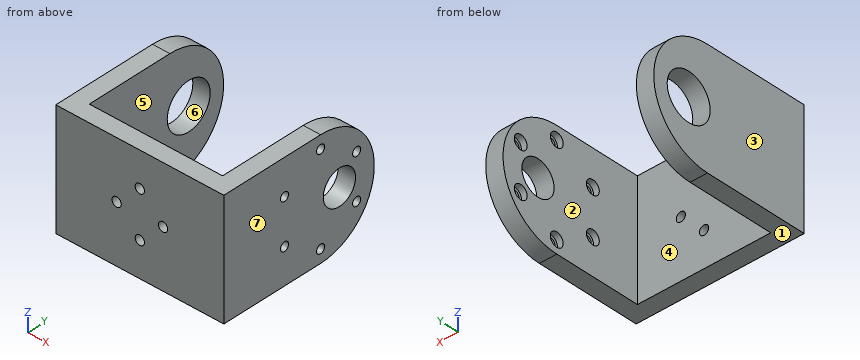
```python
from build123d import *

# Parameters (mm, degrees)
BOSS_EXTRUDE2_DEPTH         = 2
BOSS_EXTRUDE2_DEPTH_BACK    = 4
SKETCH2_W                   = 50
SKETCH2_H                   = 40
BOSS_EXTRUDE3_DEPTH         = 4
BOSS_EXTRUDE3_DEPTH_BACK    = 2
BOSS_EXTRUDE4_DEPTH         = 4
BOSS_EXTRUDE4_DEPTH_BACK    = 2
CUT_EXTRUDE1_DEPTH          = 10
CUT_EXTRUDE1_DEPTH_BACK     = 92
SKETCH7_R                   = 1.5
SKETCH7_R_2                 = 6
SKETCH8_R                   = 3
CUT_EXTRUDE2_DEPTH          = 92
Y_KSEKLIK_EKSTR_ZYON2_DEPTH = 6
SKETCH9_W                   = 11
SKETCH9_H                   = 6
BOSS_EXTRUDE5_DEPTH         = 40
SKETCH10_W                  = 7
SKETCH10_H                  = 40
CUT_EXTRUDE3_DEPTH          = 10
IZIM8_R                     = 2.395734713
KES_EKSTR_ZYON2_DEPTH       = 48
Y_KSEKLIK_EKSTR_ZYON3_DEPTH = 6
IZIM10_R                    = 8
KES_EKSTR_ZYON3_DEPTH       = 6
IZIM11_R                    = 1.6
KES_EKSTR_ZYON5_DEPTH       = 10
IZIM13_R                    = 3.884194159
Y_KSEKLIK_EKSTR_ZYON4_DEPTH = 6


with BuildPart() as part:
    # Sketch2 → Boss-Extrude2 (new, two sides: drawn at the far end of the back side and taken through both)
    with BuildSketch(Plane(origin=(0, 0, 0), x_dir=(1, 0, 0), z_dir=(0, 1, 0)).offset(-BOSS_EXTRUDE2_DEPTH_BACK)):
        with Locations((3.5, 11.198529412)):
            Rectangle(SKETCH2_W, SKETCH2_H)
    extrude(amount=BOSS_EXTRUDE2_DEPTH + BOSS_EXTRUDE2_DEPTH_BACK)

    # Sketch4 → Boss-Extrude3 (add, two sides: drawn at the far end of the back side and taken through both)
    with BuildSketch(Plane.ZY.offset(21.5).offset(-BOSS_EXTRUDE3_DEPTH_BACK)):
        with BuildLine():
            Line((8.801470588, 2), (-31.198529412, 2))
            Line((-31.198529412, 2), (-31.198529412, 32))
            ThreePointArc((-31.198529412, 32), (-11.198529412, 52), (8.801470588, 32))
            Line((8.801470588, 32), (8.801470588, 2))
        make_face()
    extrude(amount=BOSS_EXTRUDE3_DEPTH + BOSS_EXTRUDE3_DEPTH_BACK)

    # Sketch5 → Boss-Extrude4 (add, two sides: drawn at the far end of the back side and taken through both)
    with BuildSketch(Plane(origin=(28.5, 0, 0), x_dir=(0, 0, -1), z_dir=(1, 0, 0)).offset(-BOSS_EXTRUDE4_DEPTH_BACK)):
        with BuildLine():
            Line((-8.801470588, -4), (31.198529412, -4))
            Line((31.198529412, -4), (31.198529412, 32))
            ThreePointArc((31.198529412, 32), (11.198529412, 52), (-8.801470588, 32))
            Line((-8.801470588, 32), (-8.801470588, -4))
        make_face()
    extrude(amount=BOSS_EXTRUDE4_DEPTH + BOSS_EXTRUDE4_DEPTH_BACK)

    # Sketch7 → Cut-Extrude1 (cut, two sides: drawn at the far end of the back side and taken through both)
    with BuildSketch(Plane.ZY.offset(21.5).offset(-CUT_EXTRUDE1_DEPTH_BACK)):
        with Locations(Location((4.301470588, 32, 0), (0, 0, 180))):
            Circle(SKETCH7_R)
        with Locations(Location((-3.448529412, 18.576606241, 0), (0, 0, 180))):
            Circle(SKETCH7_R)
        with Locations(Location((-18.948529412, 18.576606241, 0), (0, 0, 180))):
            Circle(SKETCH7_R)
        with Locations(Location((-26.698529412, 32, 0), (0, 0, 180))):
            Circle(SKETCH7_R)
        with Locations(Location((-18.948529412, 45.423393759, 0), (0, 0, 180))):
            Circle(SKETCH7_R)
        with Locations(Location((-3.448529412, 45.423393759, 0), (0, 0, 180))):
            Circle(SKETCH7_R)
        with Locations(Location((-11.198529412, 39, 0), (0, 0, 180))):
            Circle(SKETCH7_R_2)
    extrude(amount=CUT_EXTRUDE1_DEPTH + CUT_EXTRUDE1_DEPTH_BACK, mode=Mode.SUBTRACT)

    # Sketch8 → Cut-Extrude2 (cut)
    with BuildSketch(Plane(origin=(0, 2, 0), x_dir=(1, 0, 0), z_dir=(0, 1, 0))):
        with Locations(Location((3.5, 11.198529412, 0), (0, 0, 270))):
            Circle(SKETCH8_R)
    extrude(amount=-CUT_EXTRUDE2_DEPTH, mode=Mode.SUBTRACT)

    # Çizim4 → Yükseklik-Ekstrüzyon2 (add)
    with BuildSketch(Plane(origin=(0, 2, 0), x_dir=(1, 0, 0), z_dir=(0, 1, 0))):
        with BuildLine():
            ThreePointArc((6.5, 11.198529412), (6.499830675, 11.230402947), (6.499322719, 11.262272884))
            Line((6.499322719, 11.262272884), (6, 11.262272884))
            Line((6, 11.262272884), (6, 9.540217017))
            ThreePointArc((6, 9.540217017), (6.372281323, 10.332504008), (6.5, 11.198529412))
        make_face()
        with BuildLine():
            Line((6, 11.262272884), (6.499322719, 11.262272884))
            ThreePointArc((6.499322719, 11.262272884), (6.36291811, 12.095022522), (6, 12.856841807))
            Line((6, 12.856841807), (6, 11.262272884))
        make_face()
    extrude(amount=-Y_KSEKLIK_EKSTR_ZYON2_DEPTH)

    # Sketch9 → Boss-Extrude5 (add)
    with BuildSketch(Plane(origin=(0, 0, -31.198529412), x_dir=(-1, 0, 0), z_dir=(0, 0, -1))):
        with Locations((27, -1)):
            Rectangle(SKETCH9_W, SKETCH9_H)
    extrude(amount=-BOSS_EXTRUDE5_DEPTH)

    # Sketch10 → Cut-Extrude3 (cut)
    with BuildSketch(Plane(origin=(0, 2, 0), x_dir=(1, 0, 0), z_dir=(0, 1, 0))):
        with Locations((-29, 11.198529412)):
            Rectangle(SKETCH10_W, SKETCH10_H)
    extrude(amount=-CUT_EXTRUDE3_DEPTH, mode=Mode.SUBTRACT)

    # Çizim8 → Kes-Ekstrüzyon2 (cut)
    with BuildSketch(Plane(origin=(-19.5, 0, 0), x_dir=(0, 0, -1), z_dir=(1, 0, 0))):
        with Locations((-4.301470588, 32)):
            Circle(IZIM8_R)
        with Locations((3.448529412, 45.423393759)):
            Circle(IZIM8_R)
        with Locations((18.948529412, 45.423393759)):
            Circle(IZIM8_R)
        with Locations((26.698529412, 32)):
            Circle(IZIM8_R)
        with Locations((18.948529412, 18.576606241)):
            Circle(IZIM8_R)
        with Locations((3.448529412, 18.576606241)):
            Circle(IZIM8_R)
    extrude(amount=KES_EKSTR_ZYON2_DEPTH, mode=Mode.SUBTRACT)

    # Çizim9 → Yükseklik-Ekstrüzyon3 (add)
    with BuildSketch(Plane.ZY.offset(25.5)):
        with BuildLine():
            Line((8.801470588, -4), (8.801470588, 32))
            ThreePointArc((8.801470588, 32), (-11.198529412, 52), (-31.198529412, 32))
            Line((-31.198529412, 32), (-31.198529412, -4))
            Line((-31.198529412, -4), (8.801470588, -4))
        make_face()
    extrude(amount=-Y_KSEKLIK_EKSTR_ZYON3_DEPTH)

    # Çizim10 → Kes-Ekstrüzyon3 (cut)
    with BuildSketch(Plane.ZY.offset(25.5)):
        with Locations((-11.198529412, 39)):
            Circle(IZIM10_R)
    extrude(amount=-KES_EKSTR_ZYON3_DEPTH, mode=Mode.SUBTRACT)

    # Çizim11 → Kes-Ekstrüzyon5 (cut)
    with BuildSketch(Plane.XZ.offset(4)):
        with Locations(Location((11.5, -11.198529412, 0), (0, 0, 270))):
            Circle(IZIM11_R)
        with Locations(Location((3.5, -19.198529412, 0), (0, 0, 270))):
            Circle(IZIM11_R)
        with Locations(Location((-4.5, -11.198529412, 0), (0, 0, 270))):
            Circle(IZIM11_R)
        with Locations(Location((3.5, -3.198529412, 0), (0, 0, 270))):
            Circle(IZIM11_R)
    extrude(amount=-KES_EKSTR_ZYON5_DEPTH, mode=Mode.SUBTRACT)

    # Çizim13 → Yükseklik-Ekstrüzyon4 (add)
    with BuildSketch(Plane.XZ.offset(4)):
        with Locations((3.5, -11.198529412)):
            Circle(IZIM13_R)
    extrude(amount=-Y_KSEKLIK_EKSTR_ZYON4_DEPTH)


solid = part.part
```
Geometry check sheet. Reference: the model listing, model coordinates, mm. Face numbers are marked on the shaded views. A direction names the side the tool comes from. Give positions to 0.01 mm unless a question says otherwise; leave off trailing zeros. Write each loop counter-clockwise with the first axis right and the second up, starting at its lowest first coordinate (ties: lowest second). Pieces come first, ordered by that corner, then holes.
1) Material ranges on L1, parallel to Z at x = 27.5, y = 32; L2, parallel to X at y = 20, z = 1; L3, parallel to Y at x = -6, z = -19.5, recorded low to high.
2) Gauge pin test, flat ends, axial feed: pin 1 (1.8 mm diameter, centred on y = 32, z = -26.7, fed in from +X); pin 2 (4 mm diameter, centred on x = -19.5, z = -6.5, fed in from +Y); pin 3 (3 mm diameter, centred on x = -17.5, z = -6, fed in from +Y). Record the tip position at first contact, or that the pin passes through.
3) Section check C-C, the plane y = 37.5. Record the boundary of the cut face in (x, z).
4) Section check A-A, the plane x = 11.5. Record the boundary of the cut face in (y, z), and give its area (3 significant figures).
5) Release check for a two-part mould opening along X. For the marked faces 1, 2, 3 and 4 record: pulls with the +X half, pulls with the -X half, needs draft (parallel to the pull), parting line crosses it, or undercut.
6) Access from +Z, -Z, +X, -X, +Y, -Y to the whole of each face (thin tool, end or side, straight path). Record for the marked faces 5, 6 and 7.
7) Section check D-D, the plane y = 22. Record the boundary of the cut face in (x, z), and give its area (3 significant figures).
8) Section check B-B, the plane x = 3.5. Record the boundary of the cut face in (y, z), and give its area (3 significant figures).
Computed:
1. L1: z = -31.2 to -29.09, -24.3 to 1.91, 6.7 to 8.8
1. L2: x = -25.5 to -19.5, 26.5 to 32.5
1. L3: y = -4 to 2
2. pin 1: stops at x = -19.5
2. pin 2: stops at y = 51.82
2. pin 3: stops at y = 2
3. outline: (-25.5, -30.43) - (-19.5, -30.43) - (-19.5, -19.06) - (-25.5, -19.06) - close; (-25.5, -3.34) - (-19.5, -3.34) - (-19.5, 8.03) - (-25.5, 8.03) - close; (26.5, -30.43) - (32.5, -30.43) - (32.5, -17.01) - (26.5, -17.01) - close; (26.5, -5.39) - (32.5, -5.39) - (32.5, 8.03) - (26.5, 8.03) - close
4. outline: (-4, -31.2) - (2, -31.2) - (2, -12.8) - (-4, -12.8) - close; (-4, -9.6) - (2, -9.6) - (2, 8.8) - (-4, 8.8) - close
4. area: 221 mm2
5. face 1: needs draft
5. face 2: undercut
5. face 3: pulls with the -X half
5. face 4: undercut
6. face 5: +Z, -Z, +Y
6. face 6: -X
6. face 7: +Z, -Z, +X, +Y, -Y
7. outline: (-25.5, -31.2) - (-19.5, -31.2) - (-19.5, 8.8) - (-25.5, 8.8) - close; (26.5, -31.2) - (32.5, -31.2) - (32.5, 8.8) - (26.5, 8.8) - close
7. area: 480 mm2
8. outline: (-4, -31.2) - (2, -31.2) - (2, -20.8) - (-4, -20.8) - close; (-4, -17.6) - (2, -17.6) - (2, -4.8) - (-4, -4.8) - close; (-4, -1.6) - (2, -1.6) - (2, 8.8) - (-4, 8.8) - close
8. area: 202 mm2
